Verification items for the finished model (mm, model axes). Round coordinates to 2 decimals unless told otherwise and drop trailing zeros. Loops run counter-clockwise (first coordinate to the right, second up) from the corner with the lowest first, then second, coordinate; pieces in that order, holes last. Notation, with made-up numbers: (18.5, 50) -> (55.5, 50) arc R24 ccw to (55.5, 65) -> close; hole circle Ø1 at (-1.5, 39). An arc over 180 degrees is marked (long way). Write item = value, one per line. Start each with the question number.
```python
from build123d import *

# Parameters (mm, degrees)
F1_DEPTH = 20.828


with BuildPart() as f1:
    # F0 (on Right) → F1 (new body)
    with BuildSketch(Plane.YZ):
        with BuildLine():
            ThreePointArc((-38.881893, 34.558385), (-51.67462, 46.719688), (-68.627134, 51.635321))
            ThreePointArc((-68.627134, 51.635321), (-72.794153, 29.42421), (-62.239232, 9.441939))
            ThreePointArc((-62.239232, 9.441939), (-51.458628, 2.648717), (-38.942158, 0.259733))
            ThreePointArc((-38.942158, 0.259733), (-17.433325, 7.793481), (-5.394147, 27.144075))
            ThreePointArc((-5.394147, 27.144075), (-4.710099, 31.61057), (-4.619133, 36.128227))
            ThreePointArc((-4.619133, 36.128227), (-4.249669, 39.230896), (-4.431179, 42.350209))
            ThreePointArc((-4.431179, 42.350209), (-25.860322, 57.040886), (-38.881893, 34.558385))
        make_face()
        with BuildLine():
            Line((8.578393, 32.498907), (-4.431179, 42.350209))
            ThreePointArc((-4.431179, 42.350209), (-4.249669, 39.230896), (-4.619133, 36.128227))
            ThreePointArc((-4.619133, 36.128227), (-4.710099, 31.61057), (-5.394147, 27.144075))
            Line((-5.394147, 27.144075), (8.578393, 32.498907))
        make_face()
    extrude(amount=F1_DEPTH)


solid = f1.part
```
(1) Section check C-C on z = 39. Enter the section's corners in (x, y), then the cut area to 3 significant figures.
(2) Draft check along Y on faces 1 (the flat face through (10.27, 2.16, 37.36)), 2 (the cylindrical face through (10.268, -51.459, 46.595)), 3 (the flat face through (0, -33, 29)). Enter one of: +Y half, -Y half, draft (parallel to the pull), parting line (faces both ways), or undercut.
(3) Depth check by flat-ended pin: pin 1 Ø8 at (x, y) = (18, -51) entering from -Z; pin 2 Ø8 at (x, z) = (8.5, 16) entering from +Y; pin 3 Ø2 at (y, z) = (-48.5, 14.5) entering from -X. Enter the tip coordinate at first touch or a pass-through.
(4) Section check B-B on x = 17.25. Enter the section's corners in (y, z), then the cut area to 3 significant figures.
(5) Section check A-A on z = 45. Enter the section's corners in (x, y), then the cut area to 3 significant figures.
(6) Section check D-D on y = -45. Enter the section's corners in (x, z).
(7) Scan lines: line 1 (Y direction, x = 10.25, z = 40.5); line 2 (Y direction, x = 6.5, z = 44.5); line 3 (Z direction, x = 8.75, y = -37). Record each from-to range of solid material in increasing order. Write a range as [from, to].
Computed values:
q1.outline = (0, -72.89) -> (20.83, -72.89) -> (20.83, -42.23) -> (0, -42.23) -> close; (0, -39.65) -> (20.83, -39.65) -> (20.83, -0.01) -> (0, -0.01) -> close
q1.area = 1,460 mm²
q2.face_1 = +Y half
q2.face_2 = undercut
q2.face_3 = draft
q3.pin_1 = 1.23
q3.pin_2 = -7.83
q3.pin_3 = 0
q4.outline = (-68.63, 51.64) arc R34.3 ccw to (-62.24, 9.44) arc R34.3 ccw to (-38.94, 0.26) arc R34.3 ccw to (-5.39, 27.14) -> (8.58, 32.5) -> (-4.43, 42.35) arc R17.71 ccw (long way) to (-38.88, 34.56) arc R37.29 ccw to start
q4.area = 3,030 mm²
q5.outline = (0, -71.55) -> (20.83, -71.55) -> (20.83, -48.96) -> (0, -48.96) -> close; (0, -38.87) -> (20.83, -38.87) -> (20.83, -5.03) -> (0, -5.03) -> close
q5.area = 1,180 mm²
q6.outline = (0, 0.81) -> (20.83, 0.81) -> (20.83, 41.83) -> (0, 41.83) -> close
q7.line_1 = [-72.66, -43.63], [-39.65, -1.99]
q7.line_2 = [-71.71, -48.26], [-39.02, -4.89]
q7.line_3 = [0.31, 49.11]
